```python
from build123d import *

# Parameters (mm, degrees)
F2_R     = 1.5875
F3_DEPTH = 9.525
F4_R     = 4.7625
F5_DEPTH = 9.525


with BuildPart() as f1:
    # F0 (on Front) → F1 (revolve)
    with BuildSketch(Plane.XZ):
        with BuildLine():
            add(Edge.make_bspline(
                [(2.2846506909, -40.7209396362), (21.63124053, -24.4006685783), (41.3189275658, 1.3811586384), (23.189734926, 10.8521669118), (9.2686334939, 14.001551751)],
                knots=[0, 0, 0, 0, 0.579409192, 1, 1, 1, 1], degree=3))
            Line((9.2686334939, 14.001551751), (9.2686334939, 22.7790603638))
            Line((9.2686334939, 22.7790603638), (0, 22.7790603638))
            Line((0, 22.7790603638), (0, -40.7209396362))
            Line((0, -40.7209396362), (2.2846506909, -40.7209396362))
        make_face()
    revolve(axis=Axis((0, 0, -8.9709396362), (0, 0, -1)))

    # F2 (on face) → F3 (cut)
    with BuildSketch(Plane(origin=(0, 0, -40.7209396362), x_dir=(1, 0, 0), z_dir=(0, 0, -1))):
        Circle(F2_R)
    extrude(amount=-F3_DEPTH, mode=Mode.SUBTRACT)

    # F4 (on face) → F5 (cut)
    with BuildSketch(Plane.XY.offset(22.7790603638)):
        Circle(F4_R)
    extrude(amount=-F5_DEPTH, mode=Mode.SUBTRACT)


solid = f1.part
```
Part model, mm, in its own coordinate system. A direction names the side the tool comes from. Give positions to 0.01 mm unless a question says otherwise; leave off trailing zeros. Use CSV: the item, a comma, the result in double quotes.
Item 1: Pin check, flat tips, straight feed: P1, Ø4, axis at x = 19.5, y = -7.5, coming from the -Z side; P2, Ø1.5, axis at x = 18, y = -10.5, coming from the -Z side; P3, Ø12, axis at y = -12, z = 3, coming from the +X side. Stop position of each tip, or through.
Taken from the geometry:
P1,"stops at z = -24.92"
P2,"stops at z = -23.57"
P3,"stops at x = 31.01"
Item 2: Drill centre lines: probe 1 along Y at (x, z) = (0, 16); probe 2 along Y at (x, z) = (0, -37.25); probe 3 along Z at (x, y) = (-5, 8). Where is each one in solid material? Low to high.
Taken from the geometry:
probe 1,"y = -9.27 to -4.76, 4.76 to 9.27"
probe 2,"y = -6.3 to -1.59, 1.59 to 6.3"
probe 3,"z = -34.42 to 13.96"
Item 3: Pull direction Y, two halves, no side cores. Call faces 1 (the face through (2, 0, -40.721)), 2 (the face through (0, 0, -31.196)), 3 (the face through (8.84, -2.78, 18.45)): +Y half, -Y half, draft (parallel to the pull), parting line (faces both ways), or undercut.
Taken from the geometry:
face 1,"draft"
face 2,"undercut"
face 3,"parting line"
Item 4: Which spindle directions (+Z, -Z, +X, -X, +Y, -Y) get a long thin tool onto all of the face, cutting with end or side? Do faces 4 (the face through (0, 0, 13.254)), 5 (the face through (4, 4, 22.779)), 6 (the face through (-0.34, 1.55, -36.03)). Say none if no direction does.
Taken from the geometry:
face 4,"+Z"
face 5,"+Z, +X, -X, +Y, -Y"
face 6,"-Z"
